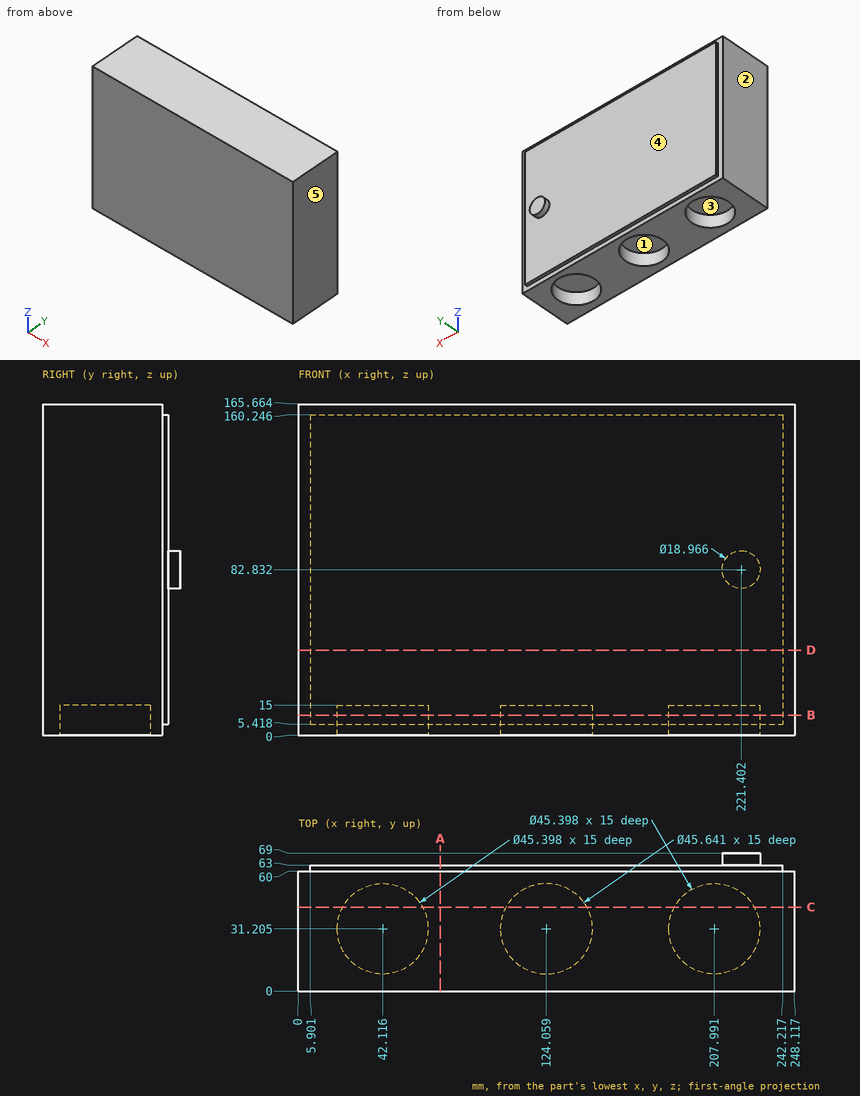
For this review, use the dimensioned drawing (mm, ordinates from the lowest corner) and the shaded views. A direction names the side the tool comes from. Round coordinates to 2 decimals unless told otherwise and drop trailing zeros. Order: outer loops, then holes, each group sorted by start corner. A loop starts at its lowest first (then second) coordinate and runs counter-clockwise, first axis right, second up. Notation, with made-up numbers: M 87,70 L 101,70 A17 cw 101,82 Z; hole C 66,-26 d5. An arc over 180 degrees is marked long. Use a Markdown table: item, result. Add a question column.
Item 1: Tool access review of the marked faces 1 and 2: name each direction out of +Z, -Z, +X, -X, +Y, -Y from which nothing blocks a thin tool from reaching the whole face with its end or side.
Item 2: Insertion check: pin 1 (12 mm diameter, centred on x = 37.5, z = 101, fed in from +Y); pin 2 (3.5 mm diameter, centred on x = 150.5, y = 62, fed in from -Z); pin 3 (0.9 mm diameter, centred on x = 153.5, y = 62, fed in from +Z). Each pin has a flat end and moves straight along its axis. Give the tip position at first contact, or say it passes through.
Item 3: Add section B-B, the plane z = 10. Give the boundary of the cut face in (x, y) (1 decimal).
Item 4: Add section D-D, the plane z = 42.5. Give the boundary of the cut face in (x, y).
Item 5: Add section A-A, the plane x = 71. Give the boundary of the cut face in (y, z) (1 decimal).
Item 6: Mouldability with a two-part tool opening along X and no side actions: class the marked faces 3, 4 and 5 as released by +X, released by -X, zero draft, split by the parting line, or undercut.
Item 7: Add section C-C, the plane y = 42. Give the boundary of the cut face in (x, z) (1 decimal).
Item 8: To check wall thickness, follow line 1 along Y through (x, z) = (224, 50.5); line 2 along X through (y, z) = (60.5, 46); line 3 along Z through (x, y) = (48.5, 45). State the ranges of each line that lie inside material, in increasing order.
Geometry results:
| question | item | result |
|---|---|---|
| 1 | face 1 | -Z |
| 1 | face 2 | +Z, -Z, -X, +Y, -Y |
| 2 | pin 1 | stops at y = 63 |
| 2 | pin 2 | stops at z = 5.42 |
| 2 | pin 3 | stops at z = 160.25 |
| 3 | outline | M 0,0 L 248.1,0 L 248.1,60 L 242.2,60 L 242.2,63 L 5.9,63 L 5.9,60 L 0,60 Z; hole C 42.1,31.2 d45.4; hole C 124.1,31.2 d45.6; hole C 208,31.2 d45.4 |
| 4 | outline | M 0,0 L 248.12,0 L 248.12,60 L 242.22,60 L 242.22,63 L 5.9,63 L 5.9,60 L 0,60 Z |
| 5 | outline | M 0,0 L 60,0 L 60,5.4 L 63,5.4 L 63,160.2 L 60,160.2 L 60,165.7 L 0,165.7 Z |
| 6 | face 3 | undercut |
| 6 | face 4 | zero draft |
| 6 | face 5 | released by +X |
| 7 | outline | M 0,0 L 22.1,0 L 22.1,15 L 62.1,15 L 62.1,0 L 104,0 L 104,15 L 144.2,15 L 144.2,0 L 188,0 L 188,15 L 228,15 L 228,0 L 248.1,0 L 248.1,165.7 L 0,165.7 Z |
| 8 | line 1 | y = 0 to 63 |
| 8 | line 2 | x = 5.9 to 242.22 |
| 8 | line 3 | z = 15 to 165.66 |
